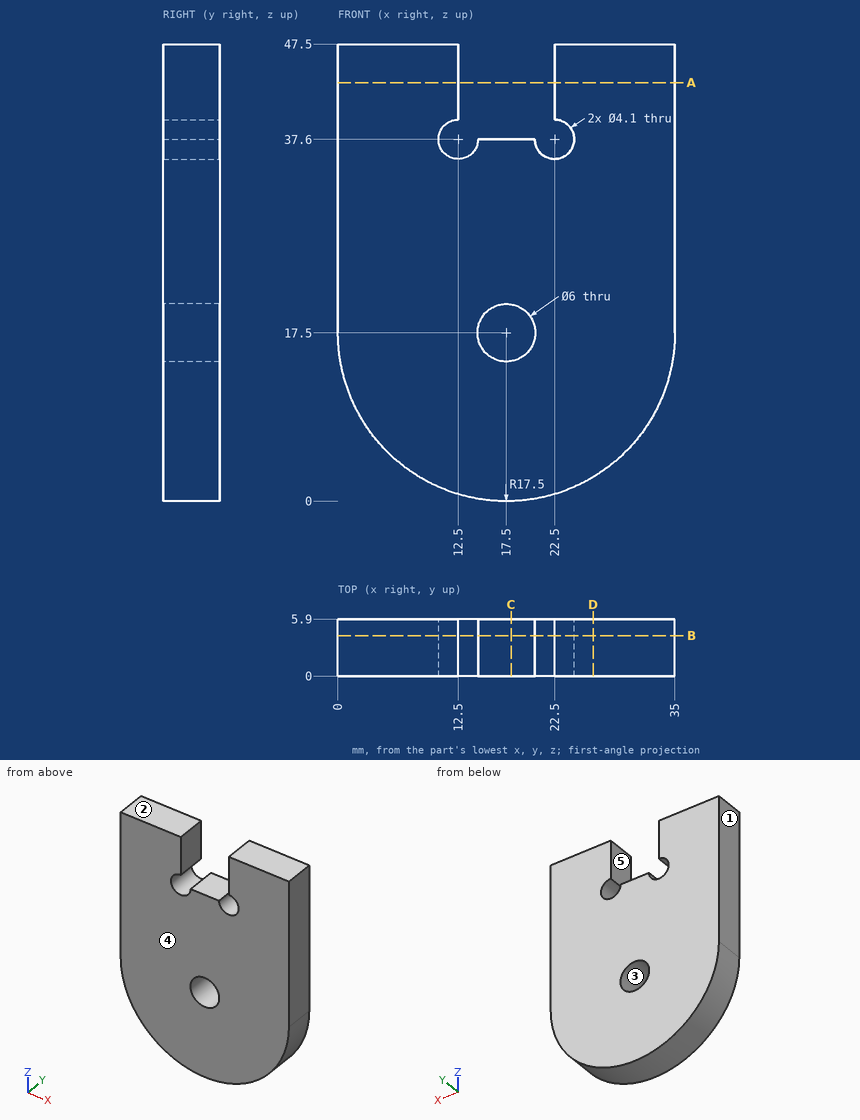
Source: three-view drawing plus pictorial views. Frame: mm from the lowest corner of the part. A direction names the side the tool comes from. Round coordinates to 2 decimals unless told otherwise and drop trailing zeros. Loops run counter-clockwise (first coordinate to the right, second up) from the corner with the lowest first, then second, coordinate; pieces in that order, holes last. Notation, with made-up numbers: (68.5, 53) - (76.5, 53) arc R15 cw to (76.5, 79) - close; hole circle Ø3 at (11, 24.5). An arc over 180 degrees is marked (long way). Write each question's results on one line, items separated by ' | '. Start each with the question number.
1) Mould query, pull axis X, two halves, no side actions, for the marked faces 1, 2 and 3. Classes: released by +X, released by -X, zero draft, split by the parting line, or undercut.
2) Cut plane C-C on x = 18. Return loops of the section in (y, z), then the cut area to 3 significant figures.
3) Cut plane D-D on x = 26.5. Return loops of the section in (y, z).
4) Access query for the marked faces 4 and 5. Directions: +Z, -Z, +X, -X, +Y, -Y. A direction counts if a zero-diameter tool reaches every point of the face in a straight line with its end or side. Return the directions, or none.
5) Cut plane A-A on z = 43.5. Return loops of the section in (x, y), then the cut area to 4 significant figures.
6) Line query: probe 1 along Z at (x, y) = (17.5, 3.3); probe 2 along X at (y, z) = (3.95, 42); probe 3 along X at (y, z) = (0.2, 36). Output: solid intervals per line, ascending. Write a range as [from, to].
7) Cut plane B-B on y = 4.2. Return loops of the section in (x, z), then the cut area to 3 significant figures.
8) First-contact query: P1, Ø1, axis at x = 13, y = 2.5, coming from the -Z side. Flat tip, straight axial feed; report the tip coordinate or a pass-through.
Verdict:
1) face 1: released by -X | face 2: zero draft | face 3: undercut
2) outline: (0, 0.01) - (5.9, 0.01) - (5.9, 14.54) - (0, 14.54) - close; (0, 20.46) - (5.9, 20.46) - (5.9, 37.6) - (0, 37.6) - close | area: 187 mm2
3) outline: (0, 2.49) - (5.9, 2.49) - (5.9, 47.5) - (0, 47.5) - close
4) face 4: +Z, -Z, +X, -X, -Y | face 5: +Z, +Y, -Y
5) outline: (0, 0) - (12.5, 0) - (12.5, 5.9) - (0, 5.9) - close; (22.5, 0) - (35, 0) - (35, 5.9) - (22.5, 5.9) - close | area: 147.5 mm2
6) probe 1: z = [0, 14.5], [20.5, 37.6] | probe 2: x = [0, 12.5], [22.5, 35] | probe 3: x = [0, 11.22], [13.78, 21.22], [23.78, 35]
7) outline: (0, 17.5) arc R17.5 ccw to (35, 17.5) - (35, 47.5) - (22.5, 47.5) - (22.5, 39.65) arc R2.05 cw (long way) to (20.45, 37.6) - (14.55, 37.6) arc R2.05 cw (long way) to (12.5, 39.65) - (12.5, 47.5) - (0, 47.5) - close; hole circle Ø6 at (17.5, 17.5) | area: 1,380 mm2
8) P1: stops at z = 0.46
